```python
from build123d import *

# Parameters (mm, degrees)
SKETCH_1_R          = 25
EXTRUDE_1_DEPTH     = 20
SKETCH_2_R          = 5
CUT_EXTRUDE_1_DEPTH = 10
SKETCH_3_R          = 10
CUT_EXTRUDE_2_DEPTH = 5
CUT_EXTRUDE_START   = -5
SKETCH_4_R          = 25
CUT_EXTRUDE_3_DEPTH = 5
EXTRUDE_START       = 5
SKETCH_5_R          = 20
SKETCH_5_R_2        = 5
EXTRUDE_2_DEPTH     = 5
SKETCH_6_R          = 3.5
EXTRUDE_3_DEPTH     = 7
SKETCH_7_R          = 6
EXTRUDE_4_DEPTH     = 12
FILLET_1_R          = 4
FILLET_2_R          = 0.5
FILLET_3_R          = 1
FILLET_4_R          = 1


with BuildPart() as part:
    # 草图1 → 凸台-拉伸1 (new body)
    with BuildSketch(Plane.XY):
        Circle(SKETCH_1_R)
    extrude(amount=EXTRUDE_1_DEPTH)

    # 草图2 → 切除-拉伸1 (cut)
    with BuildSketch(Plane.XY.offset(20)):
        Circle(SKETCH_2_R)
    extrude(amount=-CUT_EXTRUDE_1_DEPTH, mode=Mode.SUBTRACT)

    # 草图3 → 切除-拉伸2 (cut)
    with BuildSketch(Plane.XY.offset(10)):
        Circle(SKETCH_3_R)
    extrude(amount=-CUT_EXTRUDE_2_DEPTH, mode=Mode.SUBTRACT)

    # 草图4 → 切除-拉伸3 (cut)
    with BuildSketch(Plane.XY.offset(20).offset(CUT_EXTRUDE_START)):
        Circle(SKETCH_4_R)
    extrude(amount=CUT_EXTRUDE_3_DEPTH, mode=Mode.SUBTRACT)

    # 草图5 → 凸台-拉伸2 (add)
    with BuildSketch(Plane.XY.offset(15).offset(EXTRUDE_START)):
        Circle(SKETCH_5_R)
        Circle(SKETCH_5_R_2, mode=Mode.SUBTRACT)
    extrude(amount=-EXTRUDE_2_DEPTH)

    # 草图6 → 凸台-拉伸3 (add)
    with BuildSketch(Plane(origin=(24, 0, 0), x_dir=(0, 0, -1), z_dir=(1, 0, 0))):
        with Locations((-6.983226233, 0)):
            Circle(SKETCH_6_R)
    extrude(amount=EXTRUDE_3_DEPTH)

    # 草图7 → 凸台-拉伸4 (add)
    with BuildSketch(Plane(origin=(31, 0, 0), x_dir=(0, 0, -1), z_dir=(1, 0, 0))):
        with Locations((-6.983226233, 0)):
            Circle(SKETCH_7_R)
    extrude(amount=EXTRUDE_4_DEPTH)

    # 圆角1
    # the kernel refuses this fillet: 4 mm, written as the material it adds along each edge
    with BuildSketch(Plane(origin=(31, 0, 6.983226233), x_dir=(0, 0, -1), z_dir=(0, -1, 0))) as fillet_1_piece_1:
        with BuildLine():
            CenterArc((7.5, -3.708099244), FILLET_1_R, 112.024312837, 67.975687163)
            Line((3.5, -3.708099244), (3.42, -3.708099244))
            Line((3.42, -3.708099244), (3.42, 0))
            Line((3.42, 0), (3.5, 0.08))
            ThreePointArc((3.5, 0.08), (4.75, 0.08), (5.97, 0.074161985))
            Line((5.97, 0.074161985), (6, 0))
        make_face()
    revolve(axis=Axis((31, 0, 6.983226233), (1, 0, 0)))

    # 圆角2
    fillet_2_edges = [part.edges().sort_by_distance(p)[0] for p in [
        (43, 0, 12.983226233),
    ]]
    fillet(fillet_2_edges, radius=FILLET_2_R)

    # 圆角3
    fillet_3_edges = [part.edges().sort_by_distance(p)[0] for p in [
        (-25, 0, 0),
    ]]
    fillet(fillet_3_edges, radius=FILLET_3_R)

    # 圆角4
    fillet_4_edges = [part.edges().sort_by_distance(p)[0] for p in [
        (-25, 0, 15),
    ]]
    fillet(fillet_4_edges, radius=FILLET_4_R)


solid = part.part
```
Read the model definition and answer for the solid it produces. Units are mm, in the model's axes. A direction names the side the tool comes from. Give positions to 0.01 mm unless a question says otherwise; leave off trailing zeros. Write each loop counter-clockwise with the first axis right and the second up, starting at its lowest first coordinate (ties: lowest second). Pieces come first, ordered by that corner, then holes. Notation, with made-up numbers: M 16,5 L 55,5 A9 ccw 55,12 Z; hole C -34,3.25 d3. An arc over 180 degrees is marked long. Put each result on its own line as item: value. Start each with the question number.
1. The part is cut by section A-A, the plane x = 0. Give the vertices of the cut face in (y, z), and give its area (3 significant figures).
2. The part is cut by section C-C, the plane x = 28. Give the vertices of the cut face in (y, z).
3. For a pull along Z with two mould halves and no side action, classify faces 5 (the cylindrical face through (-4.336, -19.524, 17.535)), 6 (the flat face through (-5, -2, 10)), 7 (the flat face through (0, 0, 5)), 8 (the cylindrical face through (26.01, -1.34, 3.75)) as released by +Z, released by -Z, zero draft, split by the parting line, or undercut.
4. Consider line 1 along Y through (x, z) = (0, 16.5); line 2 along Z through (x, y) = (-8, 5.5); line 3 along Y through (x, z) = (0, 8.6). Determine where each line is inside the solid, lowest interval first.
5. Which of the six approach directions +Z, -Z, +X, -X, +Y, -Y give full straight-line access (tool end or side, diameter ignored) to faces 1 (the cylindrical face through (36.67, 1.8, 1.26)), 2 (the cylindrical face through (-2.17, -9.76, 7.54)), 3 (the cylindrical face through (-1.08, -4.88, 15.07)), 4 (the flat face through (0, 0, 0))?
6. Each of these flat-tipped pins is pushed along its axis until it touches: pin 1 Ø1 at (x, y) = (1.5, -0.5) entering from +Z; pin 2 Ø1.5 at (x, y) = (20.5, 15) entering from +Z; pin 3 Ø16 at (x, y) = (0, 0) entering from -Z; pin 4 Ø8 at (y, z) = (-5, 4.5) entering from -X. Where does it stop, or does it pass through?
Final values:
1. outline: M -25,1 A1 ccw -24,0 L 24,0 A1 ccw 25,1 L 25,14 A1 ccw 24,15 L 20,15 L 20,20 L 5,20 L 5,10 L 10,10 L 10,5 L -10,5 L -10,10 L -5,10 L -5,20 L -20,20 L -20,15 L -24,15 A1 ccw -25,14 Z
1. area: 749 mm²
2. outline: C 0,6.98 d7.13
3. face 5: zero draft
3. face 6: undercut
3. face 7: undercut
3. face 8: split by the parting line
4. line 1: y = -20 to -5, 5 to 20
4. line 2: z = 0 to 5, 10 to 20
4. line 3: y = -25 to -10, 10 to 25
5. face 1: +X
5. face 2: none
5. face 3: +Z
5. face 4: -Z, +X, -X, +Y, -Y
6. pin 1: stops at z = 5
6. pin 2: stops at z = 14.76
6. pin 3: stops at z = 0
6. pin 4: stops at x = -24.98
